Can you work these out from the drawing? Everything is in mm from the part's minimum corner. A direction names the side the tool comes from. Round coordinates to 2 decimals unless told otherwise and drop trailing zeros. Order: outer loops, then holes, each group sorted by start corner. A loop starts at its lowest first (then second) coordinate and runs counter-clockwise, first axis right, second up. Notation, with made-up numbers: (8, -38.75) -> (66, -38.75) arc R24 ccw to (66, -25.75) -> close; hole circle Ø4 at (66.25, 3.5). An arc over 180 degrees is marked (long way). Use a Markdown table: item, result. Add a question column.
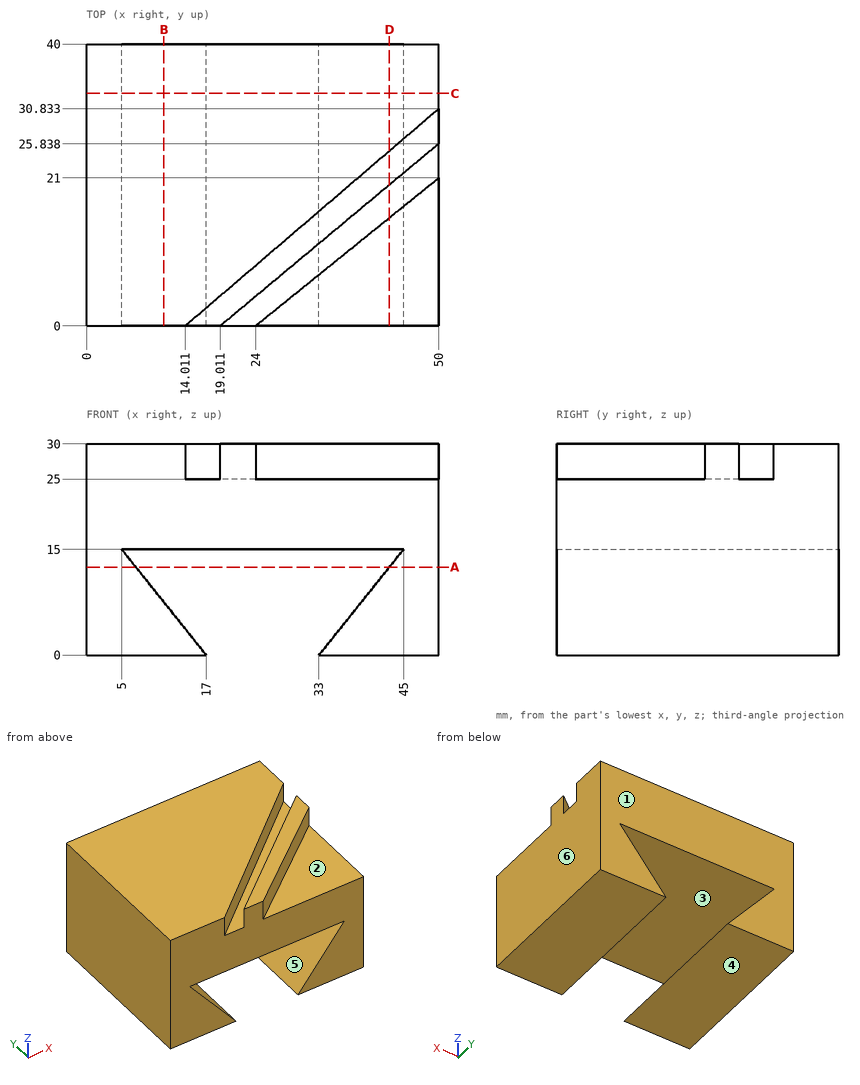
(1) I want a section at B-B on x = 11. List the corners of the cut face in (y, z) for me, and give its area (3 significant figures).
(2) I want a section at D-D on x = 43. List the corners of the cut face in (y, z) for me.
(3) I want a section at A-A on z = 12.5. List the corners of the cut face in (x, y) for me.
(4) I want a section at C-C on y = 33. List the corners of the cut face in (x, z) for me, and give its area (3 significant figures).
(5) On a 3-axis mill with a long thin cutter (end or side, diameter ignored), from which of +Z, -Z, +X, -X, +Y, -Y can I reach the whole of each face in a straight line? I mean the marked faces 1 and 2. Say none if no direction works.
(6) Please list where these lines run through material, in increasing order: probe 1 along Z at (x, y) = (34.5, 33) (1 decimal); probe 2 along X at (y, z) = (15.5, 14); probe 3 along X at (y, z) = (27, 5.25). Write a range as from..to.
(7) If we mould it in two halves opening along X, with no side actions, what happens to the marked faces 3, 4, 5 and 6? For each: pulls with the +X half, pulls with the -X half, needs draft (parallel to the pull), parting line crosses it, or undercut.
Output:
| question | item | result |
|---|---|---|
| 1 | outline | (0, 0) -> (40, 0) -> (40, 7.5) -> (0, 7.5) -> close; (0, 15) -> (40, 15) -> (40, 30) -> (0, 30) -> close |
| 1 | area | 900 mm² |
| 2 | outline | (0, 0) -> (40, 0) -> (40, 12.5) -> (0, 12.5) -> close; (0, 15) -> (40, 15) -> (40, 30) -> (24.84, 30) -> (24.84, 25) -> (20, 25) -> (20, 30) -> (15.35, 30) -> (15.35, 25) -> (0, 25) -> close |
| 3 | outline | (0, 0) -> (7, 0) -> (7, 40) -> (0, 40) -> close; (43, 0) -> (50, 0) -> (50, 40) -> (43, 40) -> close |
| 4 | outline | (0, 0) -> (17, 0) -> (5, 15) -> (45, 15) -> (33, 0) -> (50, 0) -> (50, 30) -> (0, 30) -> close |
| 4 | area | 1,080 mm² |
| 5 | face 1 | +Z, -Z, +X, -X, +Y |
| 5 | face 2 | +Z, +X, -Y |
| 6 | probe 1 | 0..1.9, 15..30 |
| 6 | probe 2 | 0..5.8, 44.2..50 |
| 6 | probe 3 | 0..12.8, 37.2..50 |
| 7 | face 3 | undercut |
| 7 | face 4 | needs draft |
| 7 | face 5 | undercut |
| 7 | face 6 | pulls with the +X half |
